Geometry check sheet. Reference: drawing and pictorial views, mm from the part's lowest x, y, z. Coordinates: 2 decimals unless noted, no trailing zeros. Loops run counter-clockwise (first coordinate to the right, second up) from the corner with the lowest first, then second, coordinate; pieces in that order, holes last. Notation, with made-up numbers: M -34.75,-16 L -16.75,-16 A26 cw -16.75,12 Z; hole C -33,81 d11. An arc over 180 degrees is marked long. Write each question's results on one line, items separated by ' | '. Start each with the question number.
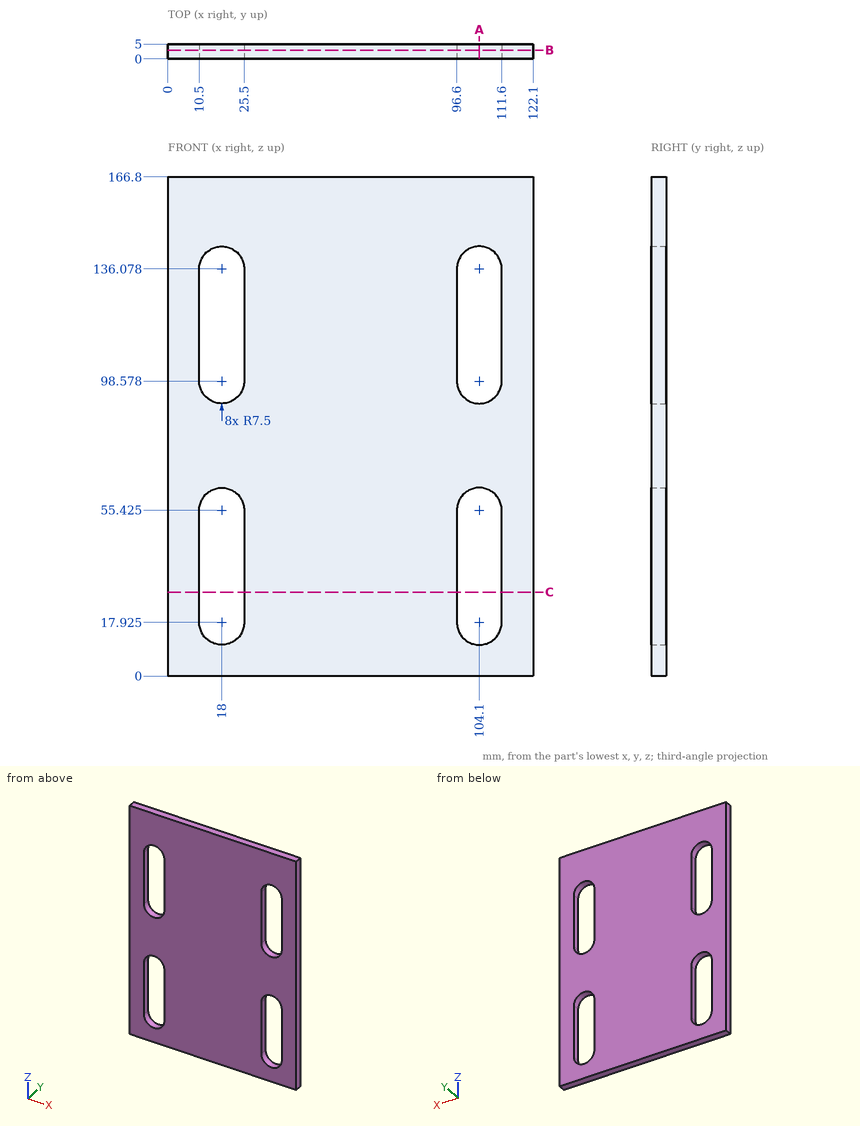
1) Gauge pin test, flat ends, axial feed: P1, Ø2.5, axis at y = 2, z = 111, coming from the -X side; P2, Ø2, axis at x = 102.5, z = 94, coming from the -Y side. Record the tip position at first contact, or that the pin passes through.
2) Section check B-B (y = 2.95). Enter the section's corners in (x, z) (1 decimal), then the cut area to 3 significant figures.
3) Thickness scan on probe 1 along X at (y, z) = (2.8, 128.5); probe 2 along X at (y, z) = (1.2, 97). Record the ranges inside material, lowest first.
4) Section check C-C (z = 28). Enter the section's corners in (x, y).
5) Section check A-A (x = 104.1). Enter the section's corners in (y, z) (1 decimal).
Return value:
1) P1: stops at x = 0 | P2: passes through
2) outline: M 0,0 L 122.1,0 L 122.1,166.8 L 0,166.8 Z; hole M 10.5,17.9 A7.5 ccw 25.5,17.9 L 25.5,55.4 A7.5 ccw 10.5,55.4 Z; hole M 10.5,98.6 A7.5 ccw 25.5,98.6 L 25.5,136.1 A7.5 ccw 10.5,136.1 Z; hole M 96.6,17.9 A7.5 ccw 111.6,17.9 L 111.6,55.4 A7.5 ccw 96.6,55.4 Z; hole M 96.6,98.6 A7.5 ccw 111.6,98.6 L 111.6,136.1 A7.5 ccw 96.6,136.1 Z | area: 17,400 mm2
3) probe 1: x = 0 to 10.5, 25.5 to 96.6, 111.6 to 122.1 | probe 2: x = 0 to 10.67, 25.33 to 96.77, 111.43 to 122.1
4) outline: M 0,0 L 10.5,0 L 10.5,5 L 0,5 Z; M 25.5,0 L 96.6,0 L 96.6,5 L 25.5,5 Z; M 111.6,0 L 122.1,0 L 122.1,5 L 111.6,5 Z
5) outline: M 0,0 L 5,0 L 5,10.4 L 0,10.4 Z; M 0,62.9 L 5,62.9 L 5,91.1 L 0,91.1 Z; M 0,143.6 L 5,143.6 L 5,166.8 L 0,166.8 Z
